from build123d import *

# Parameters (mm, degrees)
SKETCH1_W           = 342.9
SKETCH1_H           = 195.58
BOSS_EXTRUDE1_DEPTH = 7.62
SKETCH2_W           = 5.08
SKETCH2_H           = 19.05
BOSS_EXTRUDE2_DEPTH = 25.4
SKETCH3_R           = 3.048
CUT_EXTRUDE1_DEPTH  = 309.353685576
SKETCH2_4_W         = 5.08
SKETCH2_4_H         = 19.05
BOSS_EXTRUDE3_DEPTH = 44.45
SKETCH4_R           = 3.302
CUT_EXTRUDE2_DEPTH  = 299.828685576


with BuildPart() as part:
    # Sketch1 → Boss-Extrude1 (new body)
    with BuildSketch(Plane(origin=(0, 0, 0), x_dir=(1, 0, 0), z_dir=(0, 1, 0))):
        with Locations((171.45, 97.79)):
            Rectangle(SKETCH1_W, SKETCH1_H)
    extrude(amount=BOSS_EXTRUDE1_DEPTH)

    # Sketch2 → Boss-Extrude2 (add)
    with BuildSketch(Plane(origin=(0, 7.62, 0), x_dir=(1, 0, 0), z_dir=(0, 1, 0))):
        with Locations((37.086314424, 9.525)):
            Rectangle(SKETCH2_W, SKETCH2_H)
        with Locations((67.566314424, 9.525)):
            Rectangle(SKETCH2_W, SKETCH2_H)
        with Locations((153.926314424, 9.525)):
            Rectangle(SKETCH2_W, SKETCH2_H)
        with Locations((123.446314424, 9.525)):
            Rectangle(SKETCH2_W, SKETCH2_H)
    extrude(amount=BOSS_EXTRUDE2_DEPTH)

    # Sketch3 → Cut-Extrude1 (cut, through all)
    with BuildSketch(Plane.ZY.offset(-34.546314424)):
        with Locations((-9.525, 23.495)):
            Circle(SKETCH3_R)
        with BuildLine():
            Line((-19.05, 23.495), (-20.422011891, 33.02))
            Line((-20.422011891, 33.02), (2.969055393, 35.880507904))
            Line((2.969055393, 35.880507904), (0, 23.495))
            ThreePointArc((0, 23.495), (-9.525, 33.02), (-19.05, 23.495))
        make_face()
    extrude(amount=-CUT_EXTRUDE1_DEPTH, mode=Mode.SUBTRACT)

    # Sketch2<4> → Boss-Extrude3 (add)
    with BuildSketch(Plane(origin=(0, 7.62, 0), x_dir=(1, 0, 0), z_dir=(0, 1, 0))):
        with Locations((46.611314424, 186.055)):
            Rectangle(SKETCH2_4_W, SKETCH2_4_H)
        with Locations((58.041314424, 186.055)):
            Rectangle(SKETCH2_4_W, SKETCH2_4_H)
        with Locations((144.401314424, 186.055)):
            Rectangle(SKETCH2_4_W, SKETCH2_4_H)
        with Locations((132.971314424, 186.055)):
            Rectangle(SKETCH2_4_W, SKETCH2_4_H)
    extrude(amount=BOSS_EXTRUDE3_DEPTH)

    # Sketch4 → Cut-Extrude2 (cut, through all)
    with BuildSketch(Plane.ZY.offset(-44.071314424)):
        with Locations((-186.055, 42.545)):
            Circle(SKETCH4_R)
        with BuildLine():
            Line((-195.58, 42.545), (-197.59428292, 55.074082425))
            Line((-197.59428292, 55.074082425), (-172.116639762, 54.451508438))
            Line((-172.116639762, 54.451508438), (-176.53, 42.545))
            ThreePointArc((-176.53, 42.545), (-186.055, 52.07), (-195.58, 42.545))
        make_face()
    extrude(amount=-CUT_EXTRUDE2_DEPTH, mode=Mode.SUBTRACT)


solid = part.part
Source: CAD feature listing. Evaluate the final solid. Frame: model axes, mm. A direction names the side the tool comes from. Give positions to 0.01 mm unless a question says otherwise; leave off trailing zeros. Write each loop counter-clockwise with the first axis right and the second up, starting at its lowest first coordinate (ties: lowest second). Pieces come first, ordered by that corner, then holes. Notation, with made-up numbers: M 74,80 L 93,80 A7 cw 93,88 Z; hole C 80,79 d11. An arc over 180 degrees is marked long. Return JSON: item names as keys, results as strings. Group by question number.
1) Cut plane C-C, the plane z = -145. Output: boundary loops of the cut face in (x, y).
2) Pull-direction query (Z, two-part tool) for faces 1 (the face through (158, 6, 0)), 2 (the face through (58.006, 41.28, -183.005)), 3 (the face through (123.411, 33.018, -9.316)), 4 (the face through (70.106, 20, -9)); classes: pulls with the +Z half, pulls with the -Z half, needs draft (parallel to the pull), parting line crosses it, or undercut.
3) Cut plane B-B, the plane x = 117.5. Output: boundary loops of the cut face in (y, z), plus the area to 3 significant figures.
4) Cut plane A-A, the plane y = 14.5. Give the number of separate pieces and of enclosed holes in the cut face, plus the area to 3 significant figures.
5) Set-up query: faces 5 (the face through (39.626, 20, -9)), 6 (the face through (146.941, 30, -186)), 7 (the face through (44.071, 30, -186)). Return all of +Z, -Z, +X, -X, +Y, -Y with unobstructed straight access to the full face (end or side cutting, diameter ignored); none if empty.
6) Material intervals for line 1 along X through (y, z) = (32, -179); line 2 along X through (y, z) = (14, -15.5); line 3 along Y through (x, z) = (199, -84.5), sorted ascending. Write a range as [from, to].
7) Pin query (flat end, axial travel): P1, Ø4, axis at x = 143, y = 23.5, coming from the +Z side; P2, Ø15, axis at y = 15.5, z = -9.5, coming from the -X side; P3, Ø1.5, axis at x = 153.5, y = 18, coming from the -Z side; P4, Ø12, axis at x = 201, z = -25, coming from the -Y side. Return the tip coordinate at first contact, or that it passes through.
Recorded:
{
 "1": {"outline": "M 0,0 L 342.9,0 L 342.9,7.62 L 0,7.62 Z"},
 "2": {"face 1": "pulls with the +Z half", "face 2": "undercut", "face 3": "parting line crosses it", "face 4": "needs draft"},
 "3": {"outline": "M 0,-195.58 L 7.62,-195.58 L 7.62,0 L 0,0 Z", "area": "1,490 mm²"},
 "4": {"separate pieces": "8", "enclosed holes": "0", "area": "774 mm²"},
 "5": {"face 5": "+Z, -Z, +Y", "face 6": "+Z, -Z, +X, +Y", "face 7": "+Z, -Z, -X, +Y"},
 "6": {"line 1": "x = [44.07, 49.15], [55.5, 60.58], [130.43, 135.51], [141.86, 146.94]", "line 2": "x = [34.55, 39.63], [65.03, 70.11], [120.91, 125.99], [151.39, 156.47]", "line 3": "y = [0, 7.62]"},
 "7": {"P1": "stops at z = -176.53", "P2": "stops at x = 34.55", "P3": "stops at z = -19.05", "P4": "stops at y = 0"}
}
